Could you check a few things on this model? Use its own coordinates, in mm. Coordinates: 2 decimals unless noted, no trailing zeros. Write each loop counter-clockwise with the first axis right and the second up, starting at its lowest first coordinate (ties: lowest second). Pieces come first, ordered by that corner, then holes.
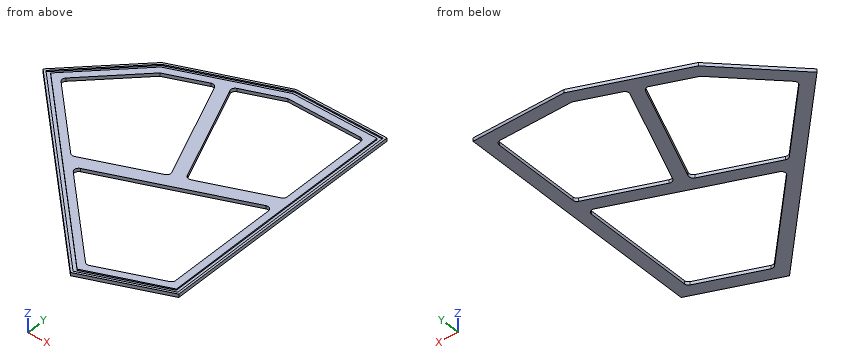
Autodesk Inventor part; units mm, degrees
ref_plane "YZ Plane" through (0, 0, 0) normal (1, 0, 0) x (0, 1, 0)
ref_plane "XZ Plane" through (0, 0, 0) normal (0, 1, 0) x (-1, 0, 0)
ref_plane "XY Plane" through (0, 0, 0) normal (0, 0, 1) x (1, 0, 0)
sketch "Sketch1" plane through (0, 0, 0) normal (0, 0, 1) x (1, 0, 0)
  line L0 (0, 273.8452) -> (193.6378, 193.6378) construction
  line L1 (193.6378, 193.6378) -> (273.8452, 0) construction
  line L2 (273.8452, 0) -> (193.6378, -193.6378) construction
  line L3 (193.6378, -193.6378) -> (0, -273.8452) construction
  line L4 (0, -273.8452) -> (-193.6378, -193.6378) construction
  line L5 (-193.6378, -193.6378) -> (-273.8452, 0) construction
  line L6 (-273.8452, 0) -> (-193.6378, 193.6378) construction
  line L7 (-193.6378, 193.6378) -> (0, 273.8452)
  line L8 (-193.6378, 193.6378) -> (0, 273.8452)
  line L9 (-459.9272, 770.6562) -> (-219.7185, 870.1539)
  line L10 (-96.8189, 233.7415) -> (-339.8229, 820.405) construction
  line L11 (-219.7185, 870.1539) -> (0, 870.1539)
  line L12 (0, 870.1539) -> (0, 273.8452)
  line L13 (-459.9272, 770.6562) -> (-615.2917, 615.2917)
  line L14 (-615.2917, 615.2917) -> (-193.6378, 193.6378)
  point P0 (0, 0)
  point P1 (0, 0)
  dimension "d0" = 506
  dimension "d2" = 260
  dimension "d3" = 635
extrude "Extrusion1" add sketch "Sketch1" along normal mid plane 8
sketch "Sketch2" plane through (0, 0, 4) normal (0, 0, 1) x (1, 0, 0)
  line L0 (-219.7185, 870.1539) -> (-459.9272, 770.6562)
  line L1 (-459.9272, 770.6562) -> (-615.2917, 615.2917)
  line L2 (-235.0492, 528.2621) -> (-412.382, 454.8085)
  line L3 (-193.6378, 193.6378) -> (0, 273.8452)
  line L4 (-96.8189, 233.7415) -> (-339.8229, 820.405) construction
  line L5 (-615.2917, 615.2917) -> (-193.6378, 193.6378)
  line L6 (-412.382, 454.8085) -> (-572.8653, 615.2917)
  line L7 (-572.8653, 615.2917) -> (-442.9336, 745.2234)
  line L8 (-442.9336, 745.2234) -> (-342.2006, 786.9484)
  line L9 (-235.0492, 528.2621) -> (-342.2006, 786.9484)
  line L10 (-207.3328, 539.7426) -> (-30, 613.1963)
  line L11 (-30, 613.1963) -> (-30, 840.1539)
  line L12 (-30, 840.1539) -> (-213.7512, 840.1539)
  line L13 (-213.7512, 840.1539) -> (-314.4842, 798.4289)
  line L14 (-207.3328, 539.7426) -> (-314.4842, 798.4289)
  line L15 (0, 273.8452) -> (0, 870.1539)
  line L16 (-412.382, 454.8085) -> (-30, 613.1963) construction
  line L17 (-389.421, 431.8474) -> (-30, 580.7245)
  line L18 (-186.5988, 229.0252) -> (-30, 293.8906)
  line L19 (-30, 293.8906) -> (-30, 580.7245)
  line L20 (-186.5988, 229.0252) -> (-389.421, 431.8474)
  point P0 (0, 0)
  dimension "d11" = 30
  dimension "d12" = 280
  dimension "d13" = 30
  dimension "d14" = 30
  dimension "d15" = 15
  dimension "d21" = 30
  dimension "d22" = 30
  dimension "d23" = 30
  dimension "d24" = 30
extrude "Extrusion2" cut sketch "Sketch2" against normal up to surface (8 mm away)
fillet "Fillet1" radius 10 12 edges at (-572.8653, 615.2917, 0) (-342.2006, 786.9484, 0) (-235.0492, 528.2621, 0) (-412.382, 454.8085, 0) (-314.4842, 798.4289, 0) (-30, 840.1539, 0) (-30, 613.1963, 0) (-207.3328, 539.7426, 0) (-389.421, 431.8474, 0) (-30, 580.7245, 0) (-30, 293.8906, 0) (-186.5988, 229.0252, 0)
sketch "Sketch4" plane through (0, 0, 4) normal (0, 0, 1) x (1, 0, 0)
  line L0 (-219.7185, 870.1539) -> (-459.9272, 770.6562)
  line L1 (0, 870.1539) -> (-219.7185, 870.1539)
  line L2 (-459.9272, 770.6562) -> (-615.2917, 615.2917)
  line L3 (-615.2917, 615.2917) -> (-193.6378, 193.6378)
  line L4 (-193.6378, 193.6378) -> (0, 273.8452)
  line L5 (0, 273.8452) -> (0, 870.1539)
  line L6 (-457.095, 766.4174) -> (-218.724, 865.1539)
  line L7 (-218.724, 865.1539) -> (-5, 865.1539)
  line L8 (-5, 865.1539) -> (-5, 277.1861)
  line L9 (-5, 277.1861) -> (-192.4647, 199.5357)
  line L10 (-192.4647, 199.5357) -> (-608.2206, 615.2917)
  line L11 (-608.2206, 615.2917) -> (-457.095, 766.4174)
  line L12 (-217.1327, 857.1539) -> (-452.5633, 759.6353)
  line L13 (-452.5633, 759.6353) -> (-596.9069, 615.2917)
  line L14 (-596.9069, 615.2917) -> (-190.5876, 208.9724)
  line L15 (-190.5876, 208.9724) -> (-13, 282.5315)
  line L16 (-13, 282.5315) -> (-13, 857.1539)
  line L17 (-13, 857.1539) -> (-217.1327, 857.1539)
  point P0 (0, 0)
  dimension "d26" = 5
  dimension "d27" = 8
extrude "Extrusion3" cut sketch "Sketch4" against normal blind 3 contours L6 L7 L8 L9 L10 L11
fillet "Fillet3" radius 16 2 edges at (-218.724, 865.1539, 2.5) (-457.095, 766.4174, 2.5)
fillet "Fillet4" radius 8 2 edges at (-452.5633, 759.6353, 2.5) (-217.1327, 857.1539, 2.5)
equation "\"d0\" = Барабан_габарит_по_кассетам"
equation "\"d2\" = Кассета_длина_грани"
equation "\"d3\" = Кассета_высота"
equation "\"d11\" = d13"
equation "\"d14\" = d13"
equation "\"d15\" = 0.5 * d13"
equation "\"d21\" = d13"
equation "\"d22\" = d13"
equation "\"d23\" = d13"
equation "\"d24\" = d13"
properties part number "ДМС 201 Внешняя рамка"
1. Please list where these lines run through material, in increasing order: line 1 along X through (y, z) = (548, 1.75); line 2 along Y through (x, z) = (-229, -2); line 3 along X through (y, z) = (818, 2.25).
Verdict:
line 1: x = -548 to -540.93, -529.62 to -505.57, -243.22 to -210.69, -187.4 to -109, -30 to -13, -5 to 0
line 2: y = 229 to 271.43, 498.3 to 592.05, 833.84 to 866.31
line 3: x = -345.63 to -332.56, -311.66 to -267.24, -30 to -13, -5 to 0
2. I want a section at A-A on x = -499. Please give me the cut outline in (y, z), plus the area to 3 significant figures.
Verdict:
outline: (499, -4) - (541.43, -4) - (541.43, 4) - (517.38, 4) - (517.38, 1) - (506.07, 1) - (506.07, 4) - (499, 4) - close; (689.16, -4) - (731.58, -4) - (731.58, 4) - (724.51, 4) - (724.51, 1) - (713.2, 1) - (713.2, 4) - (689.16, 4) - close
area: 611 mm2
3. I want a section at D-D on y = 596. Please give me the cut outline in (x, z).
Verdict:
outline: (-596, -4) - (-553.57, -4) - (-553.57, 4) - (-577.62, 4) - (-577.62, 1) - (-588.93, 1) - (-588.93, 4) - (-596, 4) - close; (-263.11, -4) - (-230.64, -4) - (-230.64, 4) - (-263.11, 4) - close; (-71.52, -4) - (0, -4) - (0, 4) - (-5, 4) - (-5, 1) - (-13, 1) - (-13, 4) - (-71.52, 4) - close
4. I want a section at B-B on z = -1. Give the number of separate pieces and of enclosed holes in the cut face, plus the area to 3 significant figures.
Verdict:
separate pieces: 1
enclosed holes: 3
area: 80,400 mm2
5. I want a section at C-C on y = 247. Please give me the cut outline in (x, z), plus the area to 3 significant figures.
Verdict:
outline: (-247, -4) - (-204.57, -4) - (-204.57, 4) - (-228.62, 4) - (-228.62, 1) - (-239.93, 1) - (-239.93, 4) - (-247, 4) - close; (-143.2, -4) - (-64.81, -4) - (-64.81, 4) - (-77.88, 4) - (-77.88, 1) - (-98.78, 1) - (-98.78, 4) - (-143.2, 4) - close
area: 870 mm2
6. For pin 1 (1.5 mm diameter, centred on x = -161.5, z = 2.5, fed in from -Y); pin 2 (4 mm diameter, centred on x = -165.5, z = -1.5, fed in from -Y); pin 3 (1.5 mm diameter, centred on y = 480, z = 3, fed in from -X), each with a flat end and sliding along its axis, tell me the tip position at first contact or that it passes through.
Verdict:
pin 1: stops at y = 206.64
pin 2: stops at y = 204.46
pin 3: stops at x = -480.75
